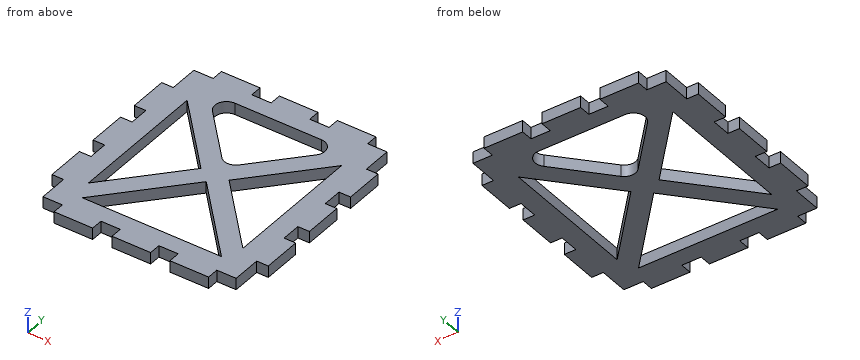
from build123d import *

# Parameters (mm, degrees)
EXTRUDE_1_DEPTH     = 3
CUT_EXTRUDE_1_DEPTH = 10
FILLET_2_R          = 3


with BuildPart() as part:
    # 草图1 → 凸台-拉伸1 (new body)
    with BuildSketch(Plane.XY):
        Polygon((-25, 27.5), (-20, 27.5), (-20, 30.5), (-10, 30.5), (-10, 27.5), (-5, 27.5), (-5, 30.5), (5, 30.5), (5, 27.5), (10, 27.5), (10, 30.5), (20, 30.5), (20, 27.5), (25, 27.5), (25, 20), (28, 20), (28, 10), (25, 10), (25, 5), (28, 5), (28, -5), (25, -5), (25, -10), (28, -10), (28, -20), (25, -20), (25, -27.5), (20, -27.5), (20, -30.5), (10, -30.5), (10, -27.5), (5, -27.5), (5, -30.5), (-5, -30.5), (-5, -27.5), (-10, -27.5), (-10, -30.5), (-20, -30.5), (-20, -27.5), (-25, -27.5), (-25, -20), (-28, -20), (-28, -10), (-25, -10), (-25, -5), (-28, -5), (-28, 5), (-25, 5), (-25, 10), (-28, 10), (-28, 20), (-25, 20), align=None)
    extrude(amount=EXTRUDE_1_DEPTH)

    # 草图2 → 切除-拉伸1 (cut)
    with BuildSketch(Plane.XY.offset(3)):
        Polygon((-18, 23), (18, 23), (0, 3.2), align=None)
        Polygon((-18, -23), (18, -23), (0, -3.2), align=None)
        Polygon((20, 18), (20, -18), (3.636363636, 0), align=None)
        Polygon((-20, 18), (-3.636363636, 0), (-20, -18), align=None)
    extrude(amount=-CUT_EXTRUDE_1_DEPTH, mode=Mode.SUBTRACT)

    # 圆角2
    fillet_2_edges = [part.edges().sort_by_distance(p)[0] for p in [
        (18, 23, 1.5),
        (0, 3.2, 1.5),
        (-18, 23, 1.5),
    ]]
    fillet(fillet_2_edges, radius=FILLET_2_R)


solid = part.part
The model under review builds one solid part; all positions refer to its coordinate system, in mm. Give positions to 0.01 mm unless a question says otherwise; leave off trailing zeros. Loops run counter-clockwise (first coordinate to the right, second up) from the corner with the lowest first, then second, coordinate; pieces in that order, holes last. Notation, with made-up numbers: (-38.5, 52.5) -> (-0.5, 52.5) arc R26 ccw to (-0.5, 66.5) -> close; hole circle Ø8 at (68.25, 39.25). An arc over 180 degrees is marked (long way). Put each result on its own line as item: value. Start each with the question number.
1. We need section C-C on y = 19. State the section outline as (x, z) points, then the cut area to 3 significant figures.
2. Clearance check with flat-ended pins moving along their axes: P1, Ø1.5, axis at x = 8.5, z = 2, coming from the -Y side; P2, Ø1.5, axis at y = -29.5, z = 1.5, coming from the +X side; P3, Ø1.5, axis at y = 29.5, z = 1.5, coming from the -X side. State where each tip first meets the part, or that it passes through.
3. Wall thickness on probe 1 along X at (y, z) = (0, 2.2); probe 2 along Y at (x, z) = (-15, 0.9); probe 3 along Y at (x, z) = (-12, 2.25): over which ranges is each line inside the solid? List them lowest first.
4. We need section B-B on y = -2.5. State the section outline as (x, z) points.
5. We need section D-D on x = -12.5. State the section outline as (y, z) points.
6. We need section A-A on x = 16. State the section outline as (y, z) points, then the cut area to 3 significant figures.
Determined:
1. outline: (-28, 0) -> (-14.05, 0) -> (-14.05, 3) -> (-28, 3) -> close; (14.05, 0) -> (28, 0) -> (28, 3) -> (14.05, 3) -> close
1. area: 83.7 mm^2
2. P1: y = -27.5
2. P2: x = 20
2. P3: x = -20
3. probe 1: -28 to -20, -3.64 to 3.64, 20 to 28
3. probe 2: -30.5 to -23, -19.7 to -12.5, 12.5 to 30.5
3. probe 3: -30.5 to -23, -16.4 to -9.2, 9.2 to 16.4, 22.9 to 30.5
4. outline: (-28, 0) -> (-20, 0) -> (-20, 3) -> (-28, 3) -> close; (-5.91, 0) -> (5.91, 0) -> (5.91, 3) -> (-5.91, 3) -> close; (20, 0) -> (28, 0) -> (28, 3) -> (20, 3) -> close
5. outline: (-30.5, 0) -> (-23, 0) -> (-23, 3) -> (-30.5, 3) -> close; (-16.95, 0) -> (-9.75, 0) -> (-9.75, 3) -> (-16.95, 3) -> close; (9.75, 0) -> (16.95, 0) -> (16.95, 3) -> (9.75, 3) -> close; (22.71, 0) -> (30.5, 0) -> (30.5, 3) -> (22.71, 3) -> close
6. outline: (-30.5, 0) -> (-23, 0) -> (-23, 3) -> (-30.5, 3) -> close; (-20.8, 0) -> (-13.6, 0) -> (-13.6, 3) -> (-20.8, 3) -> close; (13.6, 0) -> (30.5, 0) -> (30.5, 3) -> (13.6, 3) -> close
6. area: 94.8 mm^2
